```python
from build123d import *

# Parameters (mm, degrees)
SKETCH1_R          = 165
PLATE_DEPTH        = 24
SKETCH2_R          = 87.5
BEARING_HOLE_DEPTH = 235.576213628
SKETCH4_R          = 145
SKETCH4_R_2        = 140
CUT_EXTRUDE3_DEPTH = 10
SKETCH5_R          = 125
CUT_EXTRUDE4_DEPTH = 6
SKETCH6_R          = 5
CUT_EXTRUDE5_DEPTH = 235.038458378


with BuildPart() as part:
    # Sketch1 → plate (new body)
    with BuildSketch(Plane(origin=(0, 0, 0), x_dir=(1, 0, 0), z_dir=(0, 1, 0))):
        with Locations(Location((0, 0, 0), (0, 0, 270))):
            Circle(SKETCH1_R)
    extrude(amount=PLATE_DEPTH)

    # Sketch2 → bearing-hole (cut, through all)
    with BuildSketch(Plane(origin=(0, 24, 0), x_dir=(1, 0, 0), z_dir=(0, 1, 0))):
        with Locations(Location((0, 0, 0), (0, 0, 270))):
            Circle(SKETCH2_R)
    extrude(amount=-BEARING_HOLE_DEPTH, mode=Mode.SUBTRACT)

    # Sketch4 → Cut-Extrude3 (cut)
    with BuildSketch(Plane(origin=(0, 24, 0), x_dir=(1, 0, 0), z_dir=(0, 1, 0))):
        with Locations(Location((0, 0, 0), (0, 0, 270))):
            Circle(SKETCH4_R)
        with Locations(Location((0, 0, 0), (0, 0, 270))):
            Circle(SKETCH4_R_2, mode=Mode.SUBTRACT)
    extrude(amount=-CUT_EXTRUDE3_DEPTH, mode=Mode.SUBTRACT)

    # Sketch5 → Cut-Extrude4 (cut)
    with BuildSketch(Plane.XZ):
        with Locations(Location((0, 0, 0), (0, 0, 270))):
            Circle(SKETCH5_R)
    extrude(amount=-CUT_EXTRUDE4_DEPTH, mode=Mode.SUBTRACT)

    # Sketch6 → Cut-Extrude5 (cut, through all)
    with BuildSketch(Plane.XZ.offset(-6)):
        with Locations(Location((0, 105, 0), (0, 0, 270))):
            Circle(SKETCH6_R)
        with Locations(Location((74.246212025, 74.246212025, 0), (0, 0, 270))):
            Circle(SKETCH6_R)
        with Locations(Location((105, 0, 0), (0, 0, 270))):
            Circle(SKETCH6_R)
        with Locations(Location((74.246212025, -74.246212025, 0), (0, 0, 270))):
            Circle(SKETCH6_R)
        with Locations(Location((0, -105, 0), (0, 0, 270))):
            Circle(SKETCH6_R)
        with Locations(Location((-74.246212025, -74.246212025, 0), (0, 0, 270))):
            Circle(SKETCH6_R)
        with Locations(Location((-105, 0, 0), (0, 0, 270))):
            Circle(SKETCH6_R)
        with Locations(Location((-74.246212025, 74.246212025, 0), (0, 0, 270))):
            Circle(SKETCH6_R)
    extrude(amount=-CUT_EXTRUDE5_DEPTH, mode=Mode.SUBTRACT)


solid = part.part
```
Can you work these out from the model? Positions are in its coordinate system, mm. A direction names the side the tool comes from. Coordinates: 2 decimals unless noted, no trailing zeros. Order: outer loops, then holes, each group sorted by start corner. A loop starts at its lowest first (then second) coordinate and runs counter-clockwise, first axis right, second up. Notation, with made-up numbers: (70, 86.5) - (83, 86.5) arc R18 cw to (83, 120.5) - close; hole circle Ø1 at (-35, -9). An arc over 180 degrees is marked (long way). Answer in a Markdown table with one row per item.
1. Suppose I cut it at D-D (z = 105). Please give me the cut outline in (x, y), and give its area (3 significant figures).
Reply:
| item | result |
|---|---|
| outline | (-127.28, 0) - (-67.82, 0) - (-67.82, 6) - (-5, 6) - (-5, 24) - (-92.6, 24) - (-92.6, 14) - (-100, 14) - (-100, 24) - (-127.28, 24) - close; (5, 6) - (67.82, 6) - (67.82, 0) - (127.28, 0) - (127.28, 24) - (100, 24) - (100, 14) - (92.6, 14) - (92.6, 24) - (5, 24) - close |
| area | 4,970 mm^2 |
2. Suppose I cut it at C-C (y = 20). Give the number of separate pieces and of enclosed holes in the cut face, and give its area (3 significant figures).
Reply:
| item | result |
|---|---|
| separate pieces | 2 |
| enclosed holes | 10 |
| area | 56,400 mm^2 |
3. For pin 1 (11.5 mm diameter, centred on x = -74.25, z = -74.25, fed in from -Y); pin 2 (12 mm diameter, centred on x = 28, y = 21.5, fed in from +Z); pin 3 (4 mm diameter, centred on y = 17, z = 89.5, fed in from +X), each with a flat end and sliding along its axis, tell me the tip position at first contact or that it passes through.
Reply:
| item | result |
|---|---|
| pin 1 | stops at y = 6 |
| pin 2 | stops at z = 163.53 |
| pin 3 | stops at x = 139.89 |
4. If we mould it in two halves opening along Z, with no side actions, what happens to faces 1 (the cylindrical face through (-1.915, 14.874, -109.619)), 2 (the flat face through (123, 0, -25)), 3 (the cylindrical face through (-161.076, 11.832, -35.769))? For each: pulls with the +Z half, pulls with the -Z half, needs draft (parallel to the pull), parting line crosses it, or undercut.
Reply:
| item | result |
|---|---|
| face 1 | undercut |
| face 2 | needs draft |
| face 3 | parting line crosses it |
5. If I drill on line 1 along X through (y, z) = (20.5, 0); line 2 along X through (y, z) = (12.25, 0); line 3 along X through (y, z) = (16.5, -105), over which ranges is the centre line in solid material (lowest first)?
Reply:
| item | result |
|---|---|
| line 1 | x = -165 to -145, -140 to -110, -100 to -87.5, 87.5 to 100, 110 to 140, 145 to 165 |
| line 2 | x = -165 to -110, -100 to -87.5, 87.5 to 100, 110 to 165 |
| line 3 | x = -127.28 to -100, -92.6 to -5, 5 to 92.6, 100 to 127.28 |
6. Suppose I cut it at A-A (z = 0). Please give me the cut outline in (x, y), and give its area (3 significant figures).
Reply:
| item | result |
|---|---|
| outline | (-165, 0) - (-125, 0) - (-125, 6) - (-110, 6) - (-110, 24) - (-140, 24) - (-140, 14) - (-145, 14) - (-145, 24) - (-165, 24) - close; (-100, 6) - (-87.5, 6) - (-87.5, 24) - (-100, 24) - close; (87.5, 6) - (100, 6) - (100, 24) - (87.5, 24) - close; (110, 6) - (125, 6) - (125, 0) - (165, 0) - (165, 24) - (145, 24) - (145, 14) - (140, 14) - (140, 24) - (110, 24) - close |
| area | 2,810 mm^2 |
7. Suppose I cut it at B-B (x = -31). Please give me the cut outline in (y, z) (1 decimal), and give its area (3 significant figures).
Reply:
| item | result |
|---|---|
| outline | (0, -162.1) - (24, -162.1) - (24, -141.6) - (14, -141.6) - (14, -136.5) - (24, -136.5) - (24, -81.8) - (6, -81.8) - (6, -121.1) - (0, -121.1) - close; (0, 121.1) - (6, 121.1) - (6, 81.8) - (24, 81.8) - (24, 136.5) - (14, 136.5) - (14, 141.6) - (24, 141.6) - (24, 162.1) - (0, 162.1) - close |
| area | 3,280 mm^2 |
8. For faces 4 (the cylindrical face through (-79.127, 14.874, -73.162)), 5 (the flat face through (119, 14, -76)), 6 (the flat face through (85, 6, 30)), which set-ups out of +Z, -Z, +X, -X, +Y, -Y let a thin tool reach every point of the face, with its end or its side?
Reply:
| item | result |
|---|---|
| face 4 | +Y, -Y |
| face 5 | +Y |
| face 6 | -Y |
